Read the model definition and answer for the solid it produces. Units are mm, in the model's axes. A direction names the side the tool comes from. Give positions to 0.01 mm unless a question says otherwise; leave off trailing zeros. Write each loop counter-clockwise with the first axis right and the second up, starting at its lowest first coordinate (ties: lowest second). Pieces come first, ordered by that corner, then holes. Notation, with made-up numbers: (25, 18) -> (62, 18) arc R7 cw to (62, 29) -> close; hole circle Ø7 at (31.25, -38). An arc over 180 degrees is marked (long way). Write item = value, one per line.
from build123d import *

# Parameters (mm, degrees)
F0_W     = 73
F0_H     = 125
F1_DEPTH = 5
F2_D     = 2.5
F3_D     = 3.3
F4_D     = 2.5
F6_DEPTH = 25
F7_R     = 5


# Not quite as in the source:
# - a feature names something its author has since deleted; it is built from what else it names


with BuildPart() as f1:
    # F0 (on Top) → F1 (new body)
    with BuildSketch(Plane.XY):
        with Locations((-1.7126457989, 26.0309018195)):
            Rectangle(F0_W, F0_H)
    extrude(amount=F1_DEPTH)

    # F2 (through all)
    with Locations(Plane(origin=(0, 0, 0), x_dir=(1, 0, 0), z_dir=(0, 0, -1))):
        with Locations((-30.3091388196, -76.7177641392), (27.6908611804, -76.7177641392), (27.6908611804, -53.7177641392), (-30.3091388196, -53.7177641392)):
            Hole(F2_D / 2)

    # F3 (through all)
    with Locations(Plane(origin=(0, 0, 0), x_dir=(1, 0, 0), z_dir=(0, 0, -1))):
        with Locations((-21.0855398327, -47.0293052495), (-13.0855398327, -47.0293052495)):
            Hole(F3_D / 2)

    # F4 (through all)
    with Locations(Plane(origin=(0, 0, 0), x_dir=(1, 0, 0), z_dir=(0, 0, -1))):
        with Locations((-28.5, -31.9), (28.5, -31.9), (28.5, 31.9), (-28.5, 31.9)):
            Hole(F4_D / 2)

    # F5 (on face) → F6 (cut)
    with BuildSketch(Plane.XY.offset(5)):
        Polygon((24.0503107939, 35.5483236554), (7.3111363315, 52.6231595762), (-26.0799791984, 20.3202102417), (-26.0799791984, -12.9482956412), align=None)
        Polygon((29.5474557331, 26.9350063375), (-26.0799791984, -26.8796142191), (29.5474557331, -26.8796142191), align=None)
        Polygon((-3.3391041424, 52.5376833975), (23.1605084746, 78.173713526), (-26.1079283048, 78.173713526), (-26.1079283048, 52.5376833975), align=None)
    extrude(amount=-F6_DEPTH, mode=Mode.SUBTRACT)

    # F7
    f7_edges = [f1.edges().sort_by_distance(p)[0] for p in [
        (-38.212646, 88.530902, 2.5),
        (34.787354, 88.530902, 2.5),
        (34.787354, -36.469098, 2.5),
        (-38.212646, -36.469098, 2.5),
        (-26.107928, 52.537683, 2.5),
        (-26.107928, 78.173714, 2.5),
        (24.050311, 35.548324, 2.5),
        (7.311136, 52.62316, 2.5),
        (29.547456, -26.879614, 2.5),
    ]]
    fillet(f7_edges, radius=F7_R)


solid = f1.part
(1) The part is cut by section B-B on x = 16.5. Determine the outline of the cut face in (y, z).
Checks:
outline = (-36.47, 0) -> (-26.88, 0) -> (-26.88, 5) -> (-36.47, 5) -> close; (14.31, 0) -> (28.24, 0) -> (28.24, 5) -> (14.31, 5) -> close; (43.25, 0) -> (71.73, 0) -> (71.73, 5) -> (43.25, 5) -> close; (78.17, 0) -> (88.53, 0) -> (88.53, 5) -> (78.17, 5) -> close
(2) The part is cut by section D-D on y = 22.5. Determine the outline of the cut face in (x, z).
Checks:
outline = (-38.21, 0) -> (-23.83, 0) -> (-23.83, 5) -> (-38.21, 5) -> close; (10.56, 0) -> (24.96, 0) -> (24.96, 5) -> (10.56, 5) -> close; (29.55, 0) -> (34.79, 0) -> (34.79, 5) -> (29.55, 5) -> close
(3) For a pull along Y with two mould halves and no side action, classify faces 1 (the cylindrical face through (27.923, 33.009, 2.535)), 2 (the flat face through (9.73, 65.18, 2.54)), 3 (the flat face through (-10, 41, 5)), 4 (the cylindrical face through (-36.787, -34.966, 2.535)) as released by +Y, released by -Y, zero draft, split by the parting line, or undercut.
Checks:
face_1 = undercut
face_2 = undercut
face_3 = zero draft
face_4 = released by -Y
(4) A tool of negligible diameter and unlimited length cuts with its end or side. For faces 5 (the flat face through (-38.213, 25, 2)), 6 (the flat face through (-3.149, 9.235, 2.535)), from which of +Z, -Z, +X, -X, +Y, -Y can it reach the whole face along a straight path? Write none if from no direction.
Checks:
face_5 = +Z, -Z, -X, +Y, -Y
face_6 = +Z, -Z
(5) Consider L1, parallel to X at y = -31.9, z = 2.65; L2, parallel to Y at x = -28.5, z = 3.35; L3, parallel to Y at x = 15, z = 2.8. Determine where each line is inside the solid, lowest interval first.
Checks:
L1 = -38.19 to -29.75, -27.25 to 27.25, 29.75 to 34.77
L2 = -36.47 to -33.15, -30.65 to 30.65, 33.15 to 88.53
L3 = -36.47 to -26.88, 12.86 to 26.79, 44.78 to 70.28, 78.17 to 88.53
(6) The part is cut by section A-A on y = 7. Determine the outline of the cut face in (x, z).
Checks:
outline = (-38.21, 0) -> (-26.08, 0) -> (-26.08, 5) -> (-38.21, 5) -> close; (-5.46, 0) -> (8.94, 0) -> (8.94, 5) -> (-5.46, 5) -> close; (29.55, 0) -> (34.79, 0) -> (34.79, 5) -> (29.55, 5) -> close
(7) The part is cut by section C-C on z = 2.3. Count the separate pieces of the cut face and the enclosed holes in it, plus the area to 3 significant figures.
Checks:
separate_pieces = 1
enclosed_holes = 13
area = 5,260 mm²
